Autodesk Inventor part; units mm, degrees
ref_plane "YZ Plane" through (0, 0, 0) normal (1, 0, 0) x (0, 1, 0)
ref_plane "XZ Plane" through (0, 0, 0) normal (0, 1, 0) x (-1, 0, 0)
ref_plane "XY Plane" through (0, 0, 0) normal (0, 0, 1) x (1, 0, 0)
sketch "スケッチ1" plane through (0, 0, 0) normal (0, 1, 0) x (-1, 0, 0)
  circle A0 centre (0, 0) radius 15
  dimension "d0" = 30
extrude "押し出し1" add sketch "スケッチ1" along normal blind 6
sketch "スケッチ2" plane through (0, 6, 0) normal (0, 1, 0) x (1, 0, 0)
  arc A0 (2.6833, -3.1) -> (-2.6833, -3.1) centre (0, 0) ccw
  line L0 (-2.6833, -3.1) -> (2.6833, -3.1)
  point P0 (0, -3.1)
  dimension "d3" = 8.2
  dimension "d4" = 3.1
extrude "押し出し2" cut sketch "スケッチ2" against normal blind 6
sketch "スケッチ3" plane through (0, 6, 0) normal (0, 1, 0) x (1, 0, 0)
  circle A0 centre (0, 0) radius 15
  circle A1 centre (0, 0) radius 15
  line L0 (-11.1803, -10) -> (11.1803, -10)
  arc A2 (-11.1803, -10) -> (11.1803, -10) centre (0, 0) ccw
  point P0 (0, -10)
  dimension "d7" = 10
extrude "押し出し3" cut sketch "スケッチ3" against normal blind 6 contours L0 A0 picked at (2.8264, -10.7912)
sketch "スケッチ4" plane through (0, 6, 0) normal (0, 1, 0) x (1, 0, 0)
  circle A0 centre (0, 0) radius 10 construction
  point P0 (-10, 0)
  point P1 (0, 10)
  point P2 (10, 0)
  dimension "d10" = 20
hole "穴1" at (-10, 6, 0) at (0, 6, -10) at (10, 6, 0) direction (0, -1, 0) diameter 3.2 end through all
properties part number "射出_留め具1"
CAD build for the part. Positions are in the model's coordinates, mm. A direction names the side the tool comes from. Round coordinates to 2 decimals unless told otherwise and drop trailing zeros. Write each loop counter-clockwise with the first axis right and the second up, starting at its lowest first coordinate (ties: lowest second). Pieces come first, ordered by that corner, then holes. Notation, with made-up numbers: (69.25, 4) - (127.25, 4) arc R17 ccw to (127.25, 10) - close; hole circle Ø9 at (47.5, -18). An arc over 180 degrees is marked (long way). Write item = value, one per line. Start each with the question number.
Q1. Drop flat-ended pins along their axis: pin 1 (2 mm diameter, centred on y = 4, z = -9.5, fed in from +X); pin 2 (10.5 mm diameter, centred on x = 0, z = 0, fed in from -Y); pin 3 (3 mm diameter, centred on y = 4, z = -11.5, fed in from -X). Give the stop position or say it passes through.
Q2. Mould opens along X. For faces 3 (the cylindrical face through (11.56, 2.96, -0.35)), 4 (the cylindrical face through (0, 3, -15)), 5 (the flat face through (4, 6, -2)) say: pulls with the +X half, pulls with the -X half, needs draft (parallel to the pull), parting line crosses it, or undercut.
Q3. Probe L1, parallel to Z at x = 0, y = 2.25; L2, parallel to X at y = 3.7, z = 0; L3, parallel to Z at x = 10, y = 3.35. List the from-to ranges inside material, lowest first. Write a range as from..to.
Q4. Band-saw the part on B-B (x = 0). Give the cut face in (y, z).
Q5. Band-saw the part on D-D (y = 1.2). Give the cut face in (x, z).
Q6. Band-saw the part on A-A (z = 0). Give the cut face in (x, y), then the cut area to 3 significant figures.
Q7. Which spindle directions (+Z, -Z, +X, -X, +Y, -Y) get a long thin tool onto all of the face, cutting with end or side? Do faces 1 (the flat face through (0, 3, 10)), 2 (the flat face through (0, 3, 3.1)). Say none if no direction does.
Q8. Band-saw the part on C-C (x = 3.5). Give the cut face in (y, z), then the cut area to 3 significant figures.
Answers below:
q1.pin_1 = 12.36
q1.pin_2 = 0
q1.pin_3 = -11.18
q2.face_3 = undercut
q2.face_4 = parting line crosses it
q2.face_5 = needs draft
q3.L1 = -15..-11.6, -8.4..-4.1, 3.1..10
q3.L2 = -15..-11.6, -8.4..-4.1, 4.1..8.4, 11.6..15
q3.L3 = -11.18..-1.6, 1.6..10
q4.outline = (0, -15) - (6, -15) - (6, -11.6) - (0, -11.6) - close; (0, -8.4) - (6, -8.4) - (6, -4.1) - (0, -4.1) - close; (0, 3.1) - (6, 3.1) - (6, 10) - (0, 10) - close
q5.outline = (-11.18, 10) arc R15 ccw (long way) to (11.18, 10) - close; hole circle Ø3.2 at (-10, 0); hole (-2.68, 3.1) arc R4.1 ccw (long way) to (2.68, 3.1) - close; hole circle Ø3.2 at (0, -10); hole circle Ø3.2 at (10, 0)
q6.outline = (-15, 0) - (-11.6, 0) - (-11.6, 6) - (-15, 6) - close; (-8.4, 0) - (-4.1, 0) - (-4.1, 6) - (-8.4, 6) - close; (4.1, 0) - (8.4, 0) - (8.4, 6) - (4.1, 6) - close; (11.6, 0) - (15, 0) - (15, 6) - (11.6, 6) - close
q6.area = 92.4 mm2
q7.face_1 = +Z, +X, -X, +Y, -Y
q7.face_2 = +Y, -Y
q8.outline = (0, -14.59) - (6, -14.59) - (6, -2.14) - (0, -2.14) - close; (0, 2.14) - (6, 2.14) - (6, 10) - (0, 10) - close
q8.area = 122 mm2
